```python
from build123d import *

# Parameters (mm, degrees)
SKETCH1_R           = 5
SKETCH1_R_2         = 2
BOSS_EXTRUDE1_DEPTH = 2
SKETCH2_R           = 5
SKETCH2_R_2         = 2
BOSS_EXTRUDE2_DEPTH = 2
SKETCH4_R           = 3
SKETCH4_R_2         = 2.5
BOSS_EXTRUDE3_DEPTH = 46
BOSS_EXTRUDE4_DEPTH = 46
BOSS_EXTRUDE5_DEPTH = 46
SKETCH9_R           = 5
SKETCH9_R_2         = 2.5
BOSS_EXTRUDE6_DEPTH = 5


with BuildPart() as part:
    # Sketch1 → Boss-Extrude1 (new body)
    with BuildSketch(Plane.XY):
        with BuildLine():
            Line((-20, 0), (20, 0))
            Line((20, 0), (12.626516595, 30.093715997))
            ThreePointArc((12.626516595, 30.093715997), (0, 40), (-12.626516595, 30.093715997))
            Line((-12.626516595, 30.093715997), (-20, 0))
        make_face()
        with Locations((0, 20)):
            Circle(SKETCH1_R, mode=Mode.SUBTRACT)
        with Locations((0, 33)):
            Circle(SKETCH1_R_2, mode=Mode.SUBTRACT)
        with Locations((10, 8)):
            Circle(SKETCH1_R_2, mode=Mode.SUBTRACT)
        with Locations((-10, 8)):
            Circle(SKETCH1_R_2, mode=Mode.SUBTRACT)
    extrude(amount=BOSS_EXTRUDE1_DEPTH)



with BuildPart() as body_2:
    # Sketch2 → Boss-Extrude2 (new body)
    with BuildSketch(Plane(origin=(0, 0, 50), x_dir=(-1, 0, 0), z_dir=(0, 0, -1))):
        with BuildLine():
            Line((-12.626516595, 30.093715997), (-20, 0))
            Line((-20, 0), (20, 0))
            Line((20, 0), (12.626516595, 30.093715997))
            ThreePointArc((12.626516595, 30.093715997), (0, 40), (-12.626516595, 30.093715997))
        make_face()
        with Locations(Location((0, 20, 0), (0, 0, 180))):
            Circle(SKETCH2_R, mode=Mode.SUBTRACT)
        with Locations(Location((0, 33, 0), (0, 0, 180))):
            Circle(SKETCH2_R_2, mode=Mode.SUBTRACT)
        with Locations(Location((10, 8, 0), (0, 0, 180))):
            Circle(SKETCH2_R_2, mode=Mode.SUBTRACT)
        with Locations(Location((-10, 8, 0), (0, 0, 180))):
            Circle(SKETCH2_R_2, mode=Mode.SUBTRACT)
    extrude(amount=BOSS_EXTRUDE2_DEPTH)


with BuildPart() as part_1:
    add(part.part)

    add(body_2.part)  # Boss-Extrude3 merges body 2
    # Sketch4 → Boss-Extrude3 (add)
    # profile 1 of 3: a face of its own
    with BuildSketch(Plane(origin=(0, 0, 48), x_dir=(-1, 0, 0), z_dir=(0, 0, -1))):
        with Locations(Location((10, 8, 0), (0, 0, 180))):
            Circle(SKETCH4_R)
        with Locations(Location((10, 8, 0), (0, 0, 180))):
            Circle(SKETCH4_R_2, mode=Mode.SUBTRACT)
    # profile 2 of 3: a face of its own
    with BuildSketch(Plane(origin=(0, 0, 48), x_dir=(-1, 0, 0), z_dir=(0, 0, -1))):
        with Locations(Location((0, 33, 0), (0, 0, 180))):
            Circle(SKETCH4_R)
        with Locations(Location((0, 33, 0), (0, 0, 180))):
            Circle(SKETCH4_R_2, mode=Mode.SUBTRACT)
    # profile 3 of 3: a face of its own
    with BuildSketch(Plane(origin=(0, 0, 48), x_dir=(-1, 0, 0), z_dir=(0, 0, -1))):
        with Locations(Location((-10, 8, 0), (0, 0, 180))):
            Circle(SKETCH4_R)
        with Locations(Location((-10, 8, 0), (0, 0, 180))):
            Circle(SKETCH4_R_2, mode=Mode.SUBTRACT)
    extrude(amount=BOSS_EXTRUDE3_DEPTH)

    # Sketch5 → Boss-Extrude4 (add)
    with BuildSketch(Plane(origin=(0, 0, 48), x_dir=(-1, 0, 0), z_dir=(0, 0, -1))):
        Polygon((-20, 0), (20, 0), (19.019930486, 4), (-19.019930486, 4), align=None)
    extrude(amount=BOSS_EXTRUDE4_DEPTH)

    # Sketch6 → Boss-Extrude5 (add)
    with BuildSketch(Plane(origin=(0, 0, 48), x_dir=(-1, 0, 0), z_dir=(0, 0, -1))):
        Polygon((19.019930486, 4), (12.626516595, 30.093715997), (8.508199433, 30.093715997), (14.901613323, 4), align=None)
        Polygon((-19.019930486, 4), (-14.901613323, 4), (-8.508199433, 30.093715997), (-12.626516595, 30.093715997), align=None)
    extrude(amount=BOSS_EXTRUDE5_DEPTH)

    # Sketch9 → Boss-Extrude6 (add)
    # profile 1 of 4: a face of its own
    with BuildSketch(Plane.XZ):
        with Locations(Location((-10, 12.5, 0), (0, 0, 90))):
            Circle(SKETCH9_R)
        with Locations(Location((-10, 12.5, 0), (0, 0, 270))):
            Circle(SKETCH9_R_2, mode=Mode.SUBTRACT)
    # profile 2 of 4: a face of its own
    with BuildSketch(Plane.XZ):
        with Locations(Location((-10, 37.5, 0), (0, 0, 90))):
            Circle(SKETCH9_R)
        with Locations(Location((-10, 37.5, 0), (0, 0, 90))):
            Circle(SKETCH9_R_2, mode=Mode.SUBTRACT)
    # profile 3 of 4: a face of its own
    with BuildSketch(Plane.XZ):
        with Locations(Location((10, 12.5, 0), (0, 0, 90))):
            Circle(SKETCH9_R)
        with Locations(Location((10, 12.5, 0), (0, 0, 90))):
            Circle(SKETCH9_R_2, mode=Mode.SUBTRACT)
    # profile 4 of 4: a face of its own
    with BuildSketch(Plane.XZ):
        with Locations(Location((10, 37.5, 0), (0, 0, 90))):
            Circle(SKETCH9_R)
        with Locations(Location((10, 37.5, 0), (0, 0, 270))):
            Circle(SKETCH9_R_2, mode=Mode.SUBTRACT)
    extrude(amount=BOSS_EXTRUDE6_DEPTH)


solid = part_1.part
```
Verification items for the finished model (mm, model axes). A direction names the side the tool comes from. Coordinates: 2 decimals unless noted, no trailing zeros. Loops run counter-clockwise (first coordinate to the right, second up) from the corner with the lowest first, then second, coordinate; pieces in that order, holes last. Notation, with made-up numbers: (9.25, -12) -> (54.25, -12) arc R34 ccw to (54.25, 27) -> close; hole circle Ø2 at (57, 70.5). An arc over 180 degrees is marked (long way). Put each result on its own line as item: value.
1. Mould release check, pull along Y, two halves, no side actions. Record for faces 1 (the face through (-10, 0, 13)), 2 (the face through (-0.33, 30.52, 25.32)), 3 (the face through (12, -2, 11)): pulls with the +Y half, pulls with the -Y half, needs draft (parallel to the pull), parting line crosses it, or undercut.
Result set:
face 1: pulls with the -Y half
face 2: undercut
face 3: needs draft
2. Thickness scan on line 1 (X direction, y = -1.4, z = 12.5); line 2 (Y direction, x = 0, z = 49); line 3 (Z direction, x = 6, y = 10.5). Record the ranges inside material, lowest first.
Result set:
line 1: x = -15 to -12.5, -7.5 to -5, 5 to 7.5, 12.5 to 15
line 2: y = 0 to 15, 25 to 31, 35 to 40
line 3: z = 0 to 2, 48 to 50
3. Section check C-C, the plane x = 0. Give the number of separate pieces and of enclosed holes in the cut face, then the cut area to 3 significant figures.
Result set:
separate pieces: 3
enclosed holes: 0
area: 334 mm^2
4. Section check A-A, the plane z = 44.5. Record the boundary of the cut face in (x, y).
Result set:
outline: (-20, 0) -> (20, 0) -> (12.63, 30.09) -> (8.51, 30.09) -> (14.9, 4) -> (-14.9, 4) -> (-8.51, 30.09) -> (-12.63, 30.09) -> close; circle Ø6 at (-10, 8); circle Ø6 at (0, 33); circle Ø6 at (10, 8); hole circle Ø5 at (-10, 8); hole circle Ø5 at (0, 33); hole circle Ø5 at (10, 8)
5. Section check B-B, the plane y = -1. Record the boundary of the cut face in (x, z), then the cut area to 3 significant figures.
Result set:
outline: circle Ø10 at (-10, 12.5); circle Ø10 at (-10, 37.5); circle Ø10 at (10, 12.5); circle Ø10 at (10, 37.5); hole circle Ø5 at (-10, 12.5); hole circle Ø5 at (-10, 37.5); hole circle Ø5 at (10, 12.5); hole circle Ø5 at (10, 37.5)
area: 236 mm^2
6. Tool access check on faces 4 (the face through (-10, 0, 38)), 5 (the face through (-11, 10, 2)), 6 (the face through (0, 35, 49)). Record the directions out of +Z, -Z, +X, -X, +Y, -Y that give a thin tool (end or side, any length) a straight path to the whole face; none if there is none.
Result set:
face 4: -Y
face 5: none
face 6: +Z, -Z
7. Gauge pin test, flat ends, axial feed: P1, Ø6, axis at y = 31, z = 10.5, coming from the -X side; P2, Ø4, axis at x = -10, z = 37.5, coming from the +Y side; P3, Ø1.5, axis at y = 26, z = 28, coming from the +X side. Record the tip position at first contact, or that the pin passes through.
Result set:
P1: stops at x = -13.14
P2: stops at y = 30.09
P3: stops at x = 13.81
